The listing builds one solid part. Answer for the finished solid, in the listing's coordinates (mm). A direction names the side the tool comes from. Coordinates: 2 decimals unless noted, no trailing zeros. Order: outer loops, then holes, each group sorted by start corner. A loop starts at its lowest first (then second) coordinate and runs counter-clockwise, first axis right, second up. Notation, with made-up numbers: M 79,83.25 L 113,83.25 A18 ccw 113,90.25 Z; hole C 63,85.25 d7. An arc over 180 degrees is marked long. One line per item, written item: value. Start each with the question number.
Q1. Straight lines are drawn through the part: line 1 along X through (y, z) = (13, -16.5); line 2 along X through (y, z) = (18.5, 16); line 3 along X through (y, z) = (11.5, 3). For each, find the intervals that lie inside material, in ascending order. Write a range as [from, to].
Q2. Determine the mould class of faces 1 (the cylindrical face through (-58.1, 11.9, 0.2)), 2 (the flat face through (25, 18, 39.605)) for opening direction X: pulls with the +X half, pulls with the -X half, needs draft (parallel to the pull), parting line crosses it, or undercut.
Q3. Each of these flat-tipped pins is pushed along its axis until it touches: pin 1 Ø1.1 at (y, z) = (19.5, 33.5) entering from -X; pin 2 Ø2.5 at (x, z) = (2, 0.5) entering from +Y; pin 3 Ø1.5 at (x, y) = (14.5, 18.5) entering from -Z. Where does it stop, or does it pass through?
Q4. The part is cut by section A-A on y = 19.5. Give the vertices of the cut face in (x, z).
Q5. The part is cut by section C-C on z = -28. Give the vertices of the cut face in (x, y), then the cut area to 3 significant figures.
Q6. The part is cut by section D-D on z = 0. Give the vertices of the cut face in (x, y).
Q7. The part is cut by section B-B on x = 0. Give the vertices of the cut face in (y, z).
Q8. For faces 3 (the flat face through (0, 16, -47)), 4 (the cylindrical face through (-35.9, 11.9, -0.2)), 5 (the flat face through (26, 18, 42.848)), 6 (the flat face through (20, 21, 51)), determine the directions among +Z, -Z, +X, -X, +Y, -Y from which every point of the face is accessible in a straight line to the end or side of a thin tool.
```python
from build123d import *

# Parameters (mm, degrees)
SKETCH1_R           = 62.5
BOSS_EXTRUDE1_DEPTH = 21
SKETCH2_R           = 32
SKETCH2_R_2         = 6
CUT_EXTRUDE1_DEPTH  = 16
SKETCH3_R           = 6
SKETCH3_R_2         = 4
CUT_EXTRUDE2_DEPTH  = 14
SKETCH4_R           = 4
CUT_EXTRUDE3_DEPTH  = 7.5
CUT_EXTRUDE4_START  = -5
CUT_EXTRUDE4_DEPTH  = 5
CUT_EXTRUDE5_START  = -5
CUT_EXTRUDE5_DEPTH  = 5
CUT_EXTRUDE6_START  = -5
CUT_EXTRUDE6_DEPTH  = 5
CUT_EXTRUDE7_DEPTH  = 18.5


# Read off the part's stored shape, not the designer's step: Cut-Extrude6
with BuildPart() as part:
    # Sketch1 → Boss-Extrude1 (new body)
    with BuildSketch(Plane(origin=(0, 0, 0), x_dir=(1, 0, 0), z_dir=(0, 1, 0))):
        with Locations(Location((0, 0, 0), (0, 0, 90))):
            Circle(SKETCH1_R)
    extrude(amount=BOSS_EXTRUDE1_DEPTH)

    # Sketch2 → Cut-Extrude1 (cut)
    with BuildSketch(Plane(origin=(0, 21, 0), x_dir=(1, 0, 0), z_dir=(0, 1, 0))):
        with Locations(Location((0, 0, 0), (0, 0, 270))):
            Circle(SKETCH2_R)
        with Locations(Location((0, 0, 0), (0, 0, 270))):
            Circle(SKETCH2_R_2, mode=Mode.SUBTRACT)
    extrude(amount=-CUT_EXTRUDE1_DEPTH, mode=Mode.SUBTRACT)

    # Sketch3 → Cut-Extrude2 (cut)
    with BuildSketch(Plane(origin=(0, 21, 0), x_dir=(1, 0, 0), z_dir=(0, 1, 0))):
        with Locations(Location((0, 0, 0), (0, 0, 270))):
            Circle(SKETCH3_R)
        with Locations(Location((0, 0, 0), (0, 0, 270))):
            Circle(SKETCH3_R_2, mode=Mode.SUBTRACT)
    extrude(amount=-CUT_EXTRUDE2_DEPTH, mode=Mode.SUBTRACT)

    # Sketch4 → Cut-Extrude3 (cut)
    with BuildSketch(Plane(origin=(0, 21, 0), x_dir=(1, 0, 0), z_dir=(0, 1, 0))):
        with Locations(Location((0, 0, 0), (0, 0, 270))):
            Circle(SKETCH4_R)
    extrude(amount=-CUT_EXTRUDE3_DEPTH, mode=Mode.SUBTRACT)

    # Sketch5 → Cut-Extrude4 (cut)
    with BuildSketch(Plane(origin=(0, 21, 0), x_dir=(1, 0, 0), z_dir=(0, 1, 0)).offset(CUT_EXTRUDE4_START)):
        with BuildLine():
            Line((2.05, 62.466370953), (2.05, -62.466370953))
            ThreePointArc((2.05, -62.466370953), (0, -62.5), (-2.05, -62.466370953))
            Line((-2.05, -62.466370953), (-2.05, 62.466370953))
            ThreePointArc((-2.05, 62.466370953), (0, 62.5), (2.05, 62.466370953))
        make_face()
    extrude(amount=CUT_EXTRUDE4_DEPTH, mode=Mode.SUBTRACT)

    # Sketch6 → Cut-Extrude5 (cut)
    with BuildSketch(Plane(origin=(0, 21, 0), x_dir=(1, 0, 0), z_dir=(0, 1, 0)).offset(CUT_EXTRUDE5_START)):
        with BuildLine():
            Line((-48.35, -39.60463988), (48.35, -39.60463988))
            ThreePointArc((48.35, -39.60463988), (49.936833573, -37.584074456), (51.439284598, -35.5))
            Line((51.439284598, -35.5), (-51.439284598, -35.5))
            ThreePointArc((-51.439284598, -35.5), (-49.936833573, -37.584074456), (-48.35, -39.60463988))
        make_face()
    extrude(amount=CUT_EXTRUDE5_DEPTH, mode=Mode.SUBTRACT)

    # Cut-Extrude6 outline → Cut-Extrude6 (cut)
    with BuildSketch(Plane(origin=(0, 21, 0), x_dir=(1, 0, 0), z_dir=(0, 1, 0)).offset(CUT_EXTRUDE6_START)):
        with BuildLine():
            Line((6.37014237, -42.848279801), (6.37014237, -46.848279801))
            Line((6.37014237, -46.848279801), (41.37014237, -46.848279801))
            ThreePointArc((41.37014237, -46.848279801), (43.481229311, -44.895798217), (45.500273824, -42.848279801))
            Line((45.500273824, -42.848279801), (6.37014237, -42.848279801))
        make_face()
    extrude(amount=CUT_EXTRUDE6_DEPTH, mode=Mode.SUBTRACT)

    # Sketch10 → Cut-Extrude7 (cut)
    with BuildSketch(Plane(origin=(0, 21, 0), x_dir=(1, 0, 0), z_dir=(0, 1, 0))):
        with BuildLine():
            Line((-49.55, 10.803124548), (-49.55, 20))
            Line((-49.55, 20), (-44.45, 20))
            Line((-44.45, 20), (-44.45, 10.803124548))
            ThreePointArc((-44.45, 10.803124548), (-35.9, 0), (-44.45, -10.803124548))
            Line((-44.45, -10.803124548), (-44.45, -20))
            Line((-44.45, -20), (-49.55, -20))
            Line((-49.55, -20), (-49.55, -10.803124548))
            ThreePointArc((-49.55, -10.803124548), (-58.1, 0), (-49.55, 10.803124548))
        make_face()
    extrude(amount=-CUT_EXTRUDE7_DEPTH, mode=Mode.SUBTRACT)


solid = part.part
```
Output:
1. line 1: x = [-60.28, -49.55], [-44.45, -27.42], [27.42, 60.28]
1. line 2: x = [-60.42, -49.55], [-44.45, -27.71], [27.71, 60.42]
1. line 3: x = [-62.43, -57.69], [-36.31, -31.86], [-2.65, 2.65], [31.86, 62.43]
2. face 1: undercut
2. face 2: needs draft
3. pin 1: stops at x = -53.11
3. pin 2: stops at y = 13.5
3. pin 3: stops at z = -60.97
4. outline: M -51.44,35.5 A62.5 ccw -2.05,-62.47 L -2.05,-31.93 A32 cw -2.05,31.93 L -2.05,35.5 Z; M -48.35,39.6 L -2.05,39.6 L -2.05,62.47 A62.5 ccw Z; M 2.05,-62.47 A62.5 ccw 51.44,35.5 L 2.05,35.5 L 2.05,31.93 A32 cw 2.05,-31.93 Z; M 2.05,39.6 L 48.35,39.6 A62.5 ccw 45.5,42.85 L 6.37,42.85 L 6.37,46.85 L 41.37,46.85 A62.5 ccw 2.05,62.47 Z; hole M -49.55,-20 L -44.45,-20 L -44.45,-10.8 A11.1 ccw -44.45,10.8 L -44.45,20 L -49.55,20 L -49.55,10.8 A11.1 ccw -49.55,-10.8 Z
5. outline: M -55.88,0 L 55.88,0 L 55.88,21 L 15.49,21 L 15.49,5 L -15.49,5 L -15.49,21 L -55.88,21 Z
5. area: 1,850 mm^2
6. outline: M -62.5,0 L 62.5,0 L 62.5,21 L 32,21 L 32,5 L 6,5 L 6,7 L 4,7 L 4,13.5 L -4,13.5 L -4,7 L -6,7 L -6,5 L -32,5 L -32,21 L -35.9,21 L -35.9,2.5 L -58.1,2.5 L -58.1,21 L -62.5,21 Z
7. outline: M 0,-62.5 L 16,-62.5 L 16,-32 L 5,-32 L 5,-6 L 7,-6 L 7,-4 L 13.5,-4 L 13.5,4 L 7,4 L 7,6 L 5,6 L 5,32 L 16,32 L 16,62.5 L 0,62.5 Z
8. face 3: +Z, -Z, +Y
8. face 4: +Y
8. face 5: +X, +Y
8. face 6: +Z, -Z, +X, -X, +Y
